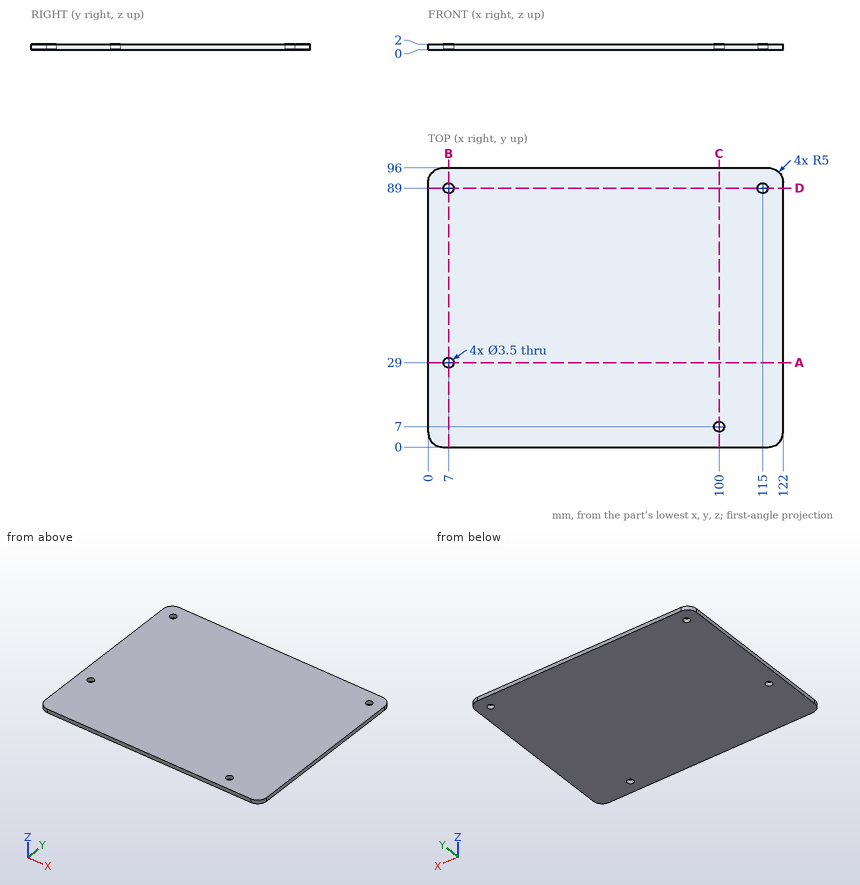
Check sheet for the drawn part. Datum: minimum x, y, z corner. Units: mm. Round coordinates to 2 decimals unless told otherwise and drop trailing zeros. Loops run counter-clockwise (first coordinate to the right, second up) from the corner with the lowest first, then second, coordinate; pieces in that order, holes last.
Item 1: Thickness scan on line 1 (X direction, y = 89, z = 1.25); line 2 (Y direction, x = 7, z = 1). Record the ranges inside material, lowest first.
Item 2: Cross-section at C-C on x = 100. Record the boundary of the cut face in (y, z).
Item 3: Cross-section at D-D on y = 89. Record the boundary of the cut face in (x, z).
Item 4: Gauge pin test, flat end, axial feed: pin 1 (3 mm diameter, centred on x = 115, y = 89, fed in from +Z). Record the tip position at first contact, or that the pin passes through.
Item 5: Cross-section at B-B on x = 7. Record the boundary of the cut face in (y, z).
Item 6: Cross-section at A-A on y = 29. Record the boundary of the cut face in (x, z), then the cut area to 3 significant figures.
Answer sheet:
1. line 1: x = 0 to 5.25, 8.75 to 113.25, 116.75 to 122
1. line 2: y = 0 to 27.25, 30.75 to 87.25, 90.75 to 96
2. outline: (0, 0) - (5.25, 0) - (5.25, 2) - (0, 2) - close; (8.75, 0) - (96, 0) - (96, 2) - (8.75, 2) - close
3. outline: (0, 0) - (5.25, 0) - (5.25, 2) - (0, 2) - close; (8.75, 0) - (113.25, 0) - (113.25, 2) - (8.75, 2) - close; (116.75, 0) - (122, 0) - (122, 2) - (116.75, 2) - close
4. pin 1: passes through
5. outline: (0, 0) - (27.25, 0) - (27.25, 2) - (0, 2) - close; (30.75, 0) - (87.25, 0) - (87.25, 2) - (30.75, 2) - close; (90.75, 0) - (96, 0) - (96, 2) - (90.75, 2) - close
6. outline: (0, 0) - (5.25, 0) - (5.25, 2) - (0, 2) - close; (8.75, 0) - (122, 0) - (122, 2) - (8.75, 2) - close
6. area: 237 mm2
